Read the model definition and answer for the solid it produces. Units are mm, in the model's axes. Round coordinates to 2 decimals unless told otherwise and drop trailing zeros. Write each loop counter-clockwise with the first axis right and the second up, starting at its lowest first coordinate (ties: lowest second). Pieces come first, ordered by that corner, then holes. Notation, with made-up numbers: (39, 71) -> (60, 71) arc R14 cw to (60, 91) -> close; hole circle Ø9 at (14, 1.25). An arc over 180 degrees is marked (long way). Return JSON: item names as keys, results as strings. Group by question number.
(1) Straight lines are drawn through the part: line 1 (Y direction, x = 133, z = 1.6); line 2 (Y direction, x = -269, z = 2.8); line 3 (X direction, y = 7.5, z = 2.85). For each, find the intervals that lie inside material, in ascending order.
(2) Given pin 1 (1.2 mm diameter, centred on x = -263, z = 2, fed in from -Y); pin 2 (1.2 mm diameter, centred on y = 4.5, z = 2.5, fed in from -X); pin 3 (1.5 mm diameter, centred on y = 2.5, z = 1.5, fed in from -X), each flat-ended and moving along its own axis, determine where each tip first touches the part or whether it passes through.
(3) A cutting plane is placed at B-B on x = -300. Give the vertices of the cut face in (y, z).
(4) A cutting plane is placed at A-A on z = 1.05. State how many separate pieces and enclosed holes the cut face has, then the cut area to 3 significant figures.
```python
from build123d import *

# Parameters (mm, degrees)
SKETCH_1_R          = 3.25
EXTRUDE_1_DEPTH     = 4
HOLE_WIZARD_M52_D   = 5.5
CUT_EXTRUDE_3_DEPTH = 353.903669576
FILLET_2_R          = 10
FILLET_3_R          = 10
HOLE_WIZARD_M31_D   = 3.4
FILLET_4_R          = 8


with BuildPart() as part:
    # Эскиз1 → Бобышка-Вытянуть1 (new body)
    with BuildSketch(Plane.XY):
        with BuildLine():
            Line((-349.818316726, 27.672449915), (-342.910885265, -16.303620822))
            Line((-342.910885265, -16.303620822), (-211.481081006, -45))
            Line((-211.481081006, -45), (211.481081006, -45))
            Line((211.481081006, -45), (342.910885265, -16.303620822))
            Line((342.910885265, -16.303620822), (349.818316726, 27.672449915))
            ThreePointArc((349.818316726, 27.672449915), (346.399852001, 39.749019149), (335, 45))
            Line((335, 45), (-335, 45))
            ThreePointArc((-335, 45), (-346.399852001, 39.749019149), (-349.818316726, 27.672449915))
        make_face()
        with Locations((-335, -10.635315981)):
            Circle(SKETCH_1_R, mode=Mode.SUBTRACT)
        with Locations(Location((335, -10.635315981, 0), (0, 0, 180))):
            Circle(SKETCH_1_R, mode=Mode.SUBTRACT)
    extrude(amount=EXTRUDE_1_DEPTH)

    # Отверстие с зазором M52 (through all)
    with Locations(Plane(origin=(0, 0, 0), x_dir=(-1, 0, 0), z_dir=(0, 0, -1))):
        with Locations((55, -6), (238.23, 10.84)):
            Hole(HOLE_WIZARD_M52_D / 2)

    # Эскиз10 → Вырез-Вытянуть3 (cut, through all)
    with BuildSketch(Plane.XY.offset(4)):
        with BuildLine():
            Line((-286.571319769, 35), (-242.571319769, 35))
            ThreePointArc((-242.571319769, 35), (-246.739453064, 3.999106889), (-245.818518827, -27.267178292))
            Line((-245.818518827, -27.267178292), (-286.571319769, -18.369213063))
            Line((-286.571319769, -18.369213063), (-286.571319769, 35))
        make_face()
        with BuildLine():
            Line((-226.671925486, 35), (-46.587816989, 35))
            Line((-46.587816989, 35), (-64.032014151, -1.707830342))
            ThreePointArc((-64.032014151, -1.707830342), (-64.961194769, -6.880112935), (-63.13950341, -11.809344562))
            Line((-63.13950341, -11.809344562), (-46.587816989, -35))
            Line((-46.587816989, -35), (-210.402090952, -35))
            Line((-210.402090952, -35), (-229.752534006, -30.775024894))
            ThreePointArc((-229.752534006, -30.775024894), (-231.306735573, 2.257420391), (-226.671925486, 35))
        make_face()
        Polygon((286.571319769, 35), (286.571319769, -18.369213063), (210.402090952, -34), (210.402090952, 35), align=None)
        Polygon((200.402090952, 35), (126.145146633, 35), (63.036502818, 22.049392771), (63.036502818, -35), (137.293447136, -35), (200.402090952, -22.049392771), align=None)
        Polygon((-29.597909048, 22.049392771), (-29.597909048, -35), (-10.072140997, -35), (53.036502818, -22.049392771), (53.036502818, 35), (33.510734767, 35), align=None)
    extrude(amount=-CUT_EXTRUDE_3_DEPTH, mode=Mode.SUBTRACT)

    # Скругление2
    fillet_2_edges = [part.edges().sort_by_distance(p)[0] for p in [
        (342.910885265, -16.303620822, 2),
        (211.481081006, -45, 2),
        (-211.481081006, -45, 2),
        (-342.910885265, -16.303620822, 2),
        (-286.571319769, -18.369213063, 2),
        (-286.571319769, 35, 2),
        (-242.571319769, 35, 2),
        (-245.818518827, -27.267178292, 2),
        (210.402090952, 35, 2),
        (286.571319769, 35, 2),
        (286.571319769, -18.369213063, 2),
        (210.402090952, -34, 2),
        (-210.402090952, -35, 2),
        (-229.752534006, -30.775024894, 2),
        (-226.671925486, 35, 2),
        (-46.587816989, 35, 2),
    ]]
    fillet(fillet_2_edges, radius=FILLET_2_R)

    # Скругление3
    fillet_3_edges = [part.edges().sort_by_distance(p)[0] for p in [
        (33.510734767, 35, 2),
        (53.036502818, 35, 2),
        (53.036502818, -22.049392771, 2),
        (-10.072140997, -35, 2),
        (-29.597909048, -35, 2),
        (-29.597909048, 22.049392771, 2),
        (63.036502818, 22.049392771, 2),
        (126.145146633, 35, 2),
        (200.402090952, 35, 2),
        (200.402090952, -22.049392771, 2),
        (137.293447136, -35, 2),
        (63.036502818, -35, 2),
    ]]
    fillet(fillet_3_edges, radius=FILLET_3_R)

    # Отверстие с зазором M31 (through all)
    with Locations(Plane.XY.offset(4)):
        with Locations((-34.597909048, 28), (-34.597909048, -27), (205.402090952, -27), (205.402090952, 28), (291.571319769, 33), (291.6163356, -2), (-291.6163356, -2), (-291.571319769, 33), (58.036502818, 28), (58.036502818, -27)):
            Hole(HOLE_WIZARD_M31_D / 2)

    # Скругление4
    fillet_4_edges = [part.edges().sort_by_distance(p)[0] for p in [
        (-46.587816989, -35, 2),
    ]]
    fillet(fillet_4_edges, radius=FILLET_4_R)


solid = part.part
```
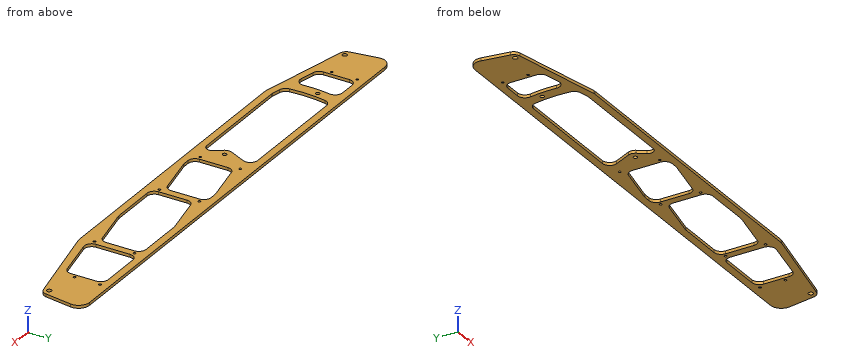
Checks:
{
 "1": {"line 1": "y = -45 to -35, 35 to 45", "line 2": "y = -32.44 to -22.21, 35 to 45", "line 3": "x = -346.65 to -286.57, -246.52 to -230.98, -59.66 to -29.6, 53.04 to 63.04, 200.4 to 210.4, 286.57 to 346.65"},
 "2": {"pin 1": "stops at y = -33.88", "pin 2": "stops at x = -346.27", "pin 3": "stops at x = -345.98"},
 "3": {"outline": "(-25.67, 0) -> (45, 0) -> (45, 4) -> (-25.67, 4) -> close"},
 "4": {"separate pieces": "1", "enclosed holes": "19", "area": "25,800 mm^2"}
}
